Geometry check sheet. Reference: the model listing, model coordinates, mm. A direction names the side the tool comes from. Give positions to 0.01 mm unless a question says otherwise; leave off trailing zeros. Order: outer loops, then holes, each group sorted by start corner. A loop starts at its lowest first (then second) coordinate and runs counter-clockwise, first axis right, second up. Notation, with made-up numbers: M -9.5,-2.75 L 46.5,-2.75 A6 cw 46.5,1.25 Z; hole C -16,27.5 d4. An arc over 180 degrees is marked long. Use CSV: the item, a comma, the result in double quotes. Start each with the question number.
from build123d import *

# Parameters (mm, degrees)
SKETCH1_W               = 50.8
SKETCH1_H               = 50.8
BOSS_EXTRUDE1_DEPTH     = 12.7
SKETCH2_R               = 3.96875
CUT_EXTRUDE1_DEPTH      = 59.198711326
F_1_4_CLEARANCE_HOLE1_D = 6.7564
SKETCH7_R               = 3.175
CUT_EXTRUDE2_DEPTH      = 6.35
F_6_CLEARANCE_HOLE1_D   = 3.7973
CUT_EXTRUDE5_START      = -1.5875
SKETCH15_R              = 3.175
CUT_EXTRUDE5_DEPTH      = 1.5875
SKETCH16_R              = 12.7
CUT_EXTRUDE6_DEPTH      = 0.127


with BuildPart() as part:
    # Sketch1 → Boss-Extrude1 (new body)
    with BuildSketch(Plane(origin=(0, 0, 0), x_dir=(1, 0, 0), z_dir=(0, 1, 0))):
        Rectangle(SKETCH1_W, SKETCH1_H)
    extrude(amount=BOSS_EXTRUDE1_DEPTH)

    # Sketch2 → Cut-Extrude1 (cut, through all)
    with BuildSketch(Plane.XY.offset(25.4)):
        with Locations((-7.9375, 0)):
            Circle(SKETCH2_R)
        with Locations((7.9375, 0)):
            Circle(SKETCH2_R)
    extrude(amount=-CUT_EXTRUDE1_DEPTH, mode=Mode.SUBTRACT)

    # 1/4 Clearance Hole1 (through all)
    with Locations(Plane(origin=(0, 12.7, 0), x_dir=(1, 0, 0), z_dir=(0, 1, 0))):
        with Locations((-19.05, -19.05), (-19.05, 19.05), (19.05, 19.05), (19.05, -19.05)):
            Hole(F_1_4_CLEARANCE_HOLE1_D / 2)

    # Sketch7 → Cut-Extrude2 (cut)
    with BuildSketch(Plane(origin=(0, 12.7, 0), x_dir=(1, 0, 0), z_dir=(0, 1, 0))):
        with Locations(Location((-16.51, 0, 0), (0, 0, 270))):
            Circle(SKETCH7_R)
        with Locations(Location((0, 16.51, 0), (0, 0, 270))):
            Circle(SKETCH7_R)
        with Locations(Location((16.51, 0, 0), (0, 0, 270))):
            Circle(SKETCH7_R)
        with Locations(Location((0, -16.51, 0), (0, 0, 270))):
            Circle(SKETCH7_R)
    extrude(amount=-CUT_EXTRUDE2_DEPTH, mode=Mode.SUBTRACT)

    # #6 Clearance Hole1 (through all)
    with Locations(Plane(origin=(0, 6.35, 0), x_dir=(1, 0, 0), z_dir=(0, 1, 0))):
        with Locations((-16.51, 0), (0, 16.51), (16.51, 0), (0, -16.51)):
            Hole(F_6_CLEARANCE_HOLE1_D / 2)

    # Sketch15 → Cut-Extrude5 (cut)
    with BuildSketch(Plane.XZ.offset(CUT_EXTRUDE5_START)):
        with Locations(Location((0, 16.51, 0), (0, 0, 90))):
            Circle(SKETCH15_R)
        with Locations(Location((16.51, 0, 0), (0, 0, 90))):
            Circle(SKETCH15_R)
        with Locations(Location((0, -16.51, 0), (0, 0, 90))):
            Circle(SKETCH15_R)
        with Locations(Location((-16.51, 0, 0), (0, 0, 90))):
            Circle(SKETCH15_R)
    extrude(amount=CUT_EXTRUDE5_DEPTH, mode=Mode.SUBTRACT)

    # Sketch16 → Cut-Extrude6 (cut)
    with BuildSketch(Plane(origin=(0, 12.7, 0), x_dir=(1, 0, 0), z_dir=(0, 1, 0))):
        with Locations(Location((0, 0, 0), (0, 0, 270))):
            Circle(SKETCH16_R)
    extrude(amount=-CUT_EXTRUDE6_DEPTH, mode=Mode.SUBTRACT)


solid = part.part
(1) Access from +Z, -Z, +X, -X, +Y, -Y to the whole of each face (thin tool, end or side, straight path). Record for faces 5 (the face through (1.93, 0.8, 13.99)), 6 (the face through (17, 6.35, 2)), 7 (the face through (0.2, 3.9, -18.4)).
(2) Sectioned sample at A-A on y = 3. Give the number of separate pieces and of enclosed holes in the cut face, then the cut area to 3 significant figures.
(3) Thickness scan on line 1 (X direction, y = 9, z = -19.05) (3 decimals); line 2 (X direction, y = 10.25, z = 0) (3 decimals); line 3 (Z direction, x = -19.05, y = 3.25). Record the ranges inside material, lowest first.
(4) Sectioned sample at B-B on z = -21.5. Record the cut outline in (x, y).
(5) Go/stop test with flat-tipped pins: P1, Ø1.5, axis at x = 7.5, z = 6.5, coming from the +Y side; P2, Ø5, axis at x = 18, z = -0.5, coming from the -Y side; P3, Ø1, axis at x = -6, z = 3, coming from the -Y side; P4, Ø5, axis at x = 16.51, z = 0, coming from the +Y side. Record where each tip stops, or that it passes through.
(6) Draft check along X on faces 1 (the face through (0, 0, 0)), 2 (the face through (-2, 6.35, 16)), 3 (the face through (2, 1.588, 16)), 4 (the face through (-25.4, 6, 0)). Enter one of: +X half, -X half, draft (parallel to the pull), parting line (faces both ways), or undercut.
Responses:
1,face 5,"-Y"
1,face 6,"+Y"
1,face 7,"+Y, -Y"
2,separate pieces,"3"
2,enclosed holes,"8"
2,area,"1,860 mm2"
3,line 1,"-25.4 to -22.428, -15.672 to -1.905, 1.905 to 15.672, 22.428 to 25.4"
3,line 2,"-25.4 to -19.685, -13.335 to 13.335, 19.685 to 25.4"
3,line 3,"-25.4 to -22.43, -15.67 to 15.67, 22.43 to 25.4"
4,outline,"M -25.4,0 L -21.38,0 L -21.38,12.7 L -25.4,12.7 Z; M -16.72,0 L -11.91,0 A3.97 cw -3.97,0 L 3.97,0 A3.97 cw 11.91,0 L 16.72,0 L 16.72,12.7 L -16.72,12.7 Z; M 21.38,0 L 25.4,0 L 25.4,12.7 L 21.38,12.7 Z"
5,P1,"y = 12.57"
5,P2,"y = 0"
5,P3,"y = 3.13"
5,P4,"y = 6.35"
6,face 1,"draft"
6,face 2,"undercut"
6,face 3,"undercut"
6,face 4,"-X half"
